Could you check a few things on this drawing? It's one solid part, dimensions in mm from its lowest x, y, z. A direction names the side the tool comes from. Give positions to 0.01 mm unless a question says otherwise; leave off trailing zeros. Loops run counter-clockwise (first coordinate to the right, second up) from the corner with the lowest first, then second, coordinate; pieces in that order, holes last. Notation, with made-up numbers: (-2.75, 85) - (36.25, 85) arc R14 ccw to (36.25, 90) - close; hole circle Ø9 at (69, -24.5). An arc over 180 degrees is marked (long way). Use a Markdown table: item, result.
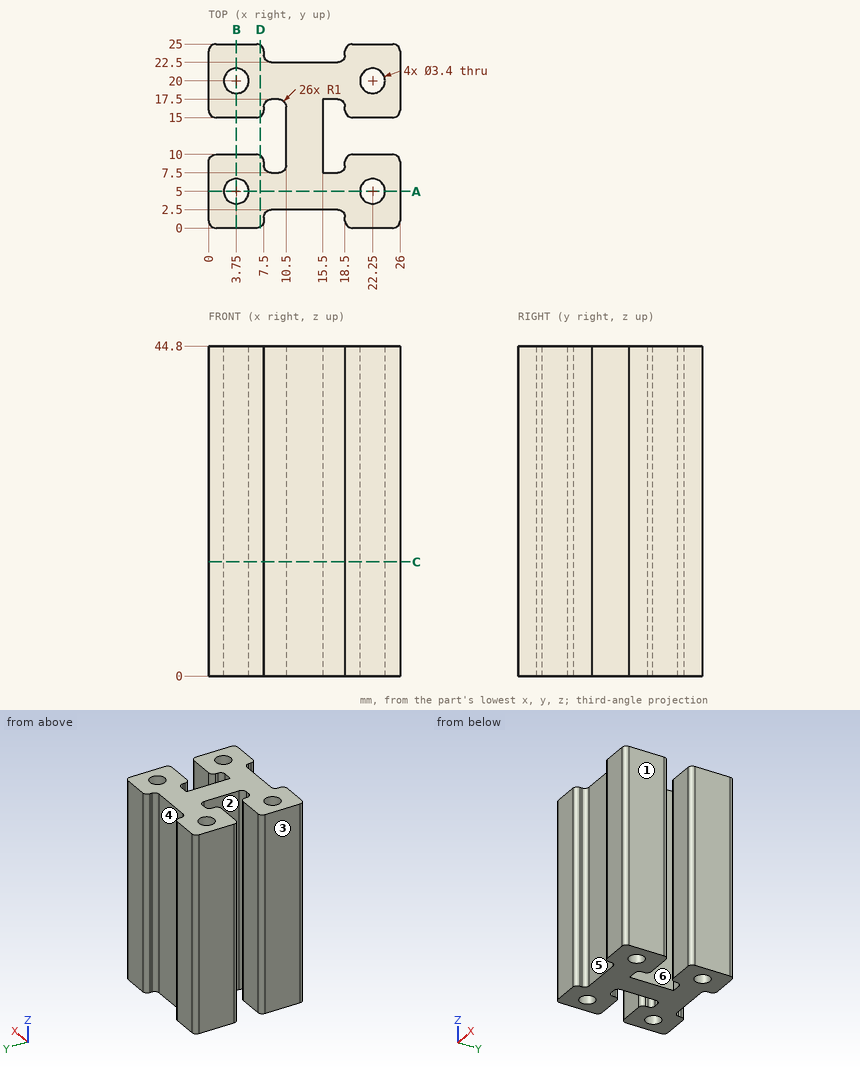
(1) If I drill on line 1 (Y direction, x = 3.75, z = 17); line 2 (X direction, y = 5, z = 18.5); line 3 (X direction, y = 8.5, z = 7), over which ranges is the centre line in solid material (lowest first)?
A:
| item | result |
|---|---|
| line 1 | 0 to 3.3, 6.7 to 10, 15 to 18.3, 21.7 to 25 |
| line 2 | 0 to 2.05, 5.45 to 20.55, 23.95 to 26 |
| line 3 | 0 to 7.5, 10.5 to 15.5, 18.5 to 26 |
(2) Will these pins go through, and if not, where does the flat tip stop? pin 1 (6 mm diameter, centred on x = 21.5, y = 22, fed in from -Z); pin 2 (2.5 mm diameter, centred on x = 15, z = 29, fed in from +Y); pin 3 (1.5 mm diameter, centred on x = 11.5, z = 28.5, fed in from -Y); pin 4 (1.5 mm diameter, centred on y = 13.5, z = 13, fed in from +X).
A:
| item | result |
|---|---|
| pin 1 | z = 0 |
| pin 2 | y = 22.5 |
| pin 3 | y = 2.5 |
| pin 4 | x = 15.5 |
(3) We'd pull the mould along X, two halves only. Please class the marked faces 1, 2 and 3: pulls with the +X half, pulls with the -X half, needs draft (parallel to the pull), parting line crosses it, or undercut.
A:
| item | result |
|---|---|
| face 1 | pulls with the +X half |
| face 2 | undercut |
| face 3 | pulls with the -X half |
(4) Suppose I cut it at C-C on z = 15.5. Count the separate pieces of the cut face and the enclosed holes in it, plus the area to 3 significant figures.
A:
| item | result |
|---|---|
| separate pieces | 1 |
| enclosed holes | 4 |
| area | 422 mm2 |
(5) Suppose I cut it at A-A on y = 5. Write out the boundary of the cut face in (x, z).
A:
| item | result |
|---|---|
| outline | (0, 0) - (2.05, 0) - (2.05, 44.8) - (0, 44.8) - close; (5.45, 0) - (20.55, 0) - (20.55, 44.8) - (5.45, 44.8) - close; (23.95, 0) - (26, 0) - (26, 44.8) - (23.95, 44.8) - close |
(6) Suppose I cut it at B-B on x = 3.75. Write out the boundary of the cut face in (y, z).
A:
| item | result |
|---|---|
| outline | (0, 0) - (3.3, 0) - (3.3, 44.8) - (0, 44.8) - close; (6.7, 0) - (10, 0) - (10, 44.8) - (6.7, 44.8) - close; (15, 0) - (18.3, 0) - (18.3, 44.8) - (15, 44.8) - close; (21.7, 0) - (25, 0) - (25, 44.8) - (21.7, 44.8) - close |
(7) Suppose I cut it at D-D on x = 7. Write out the boundary of the cut face in (y, z), plus the area to 3 significant figures.
A:
| item | result |
|---|---|
| outline | (0.13, 0) - (9.87, 0) - (9.87, 44.8) - (0.13, 44.8) - close; (15.13, 0) - (24.87, 0) - (24.87, 44.8) - (15.13, 44.8) - close |
| area | 872 mm2 |
(8) On a 3-axis mill with a long thin cutter (end or side, diameter ignored), from which of +Z, -Z, +X, -X, +Y, -Y can I reach the whole of each face in a straight line? I mean the marked faces 4, 5 and 6. Say none if no direction works.
A:
| item | result |
|---|---|
| face 4 | +Z, -Z, +Y |
| face 5 | +Z, -Z, -Y |
| face 6 | +Z, -Z |
